Can you work these out from the model? Positions are in its coordinate system, mm. Give positions to 0.01 mm unless a question says otherwise; leave off trailing zeros. Loops run counter-clockwise (first coordinate to the right, second up) from the corner with the lowest first, then second, coordinate; pieces in that order, holes last. Notation, with made-up numbers: M 25.5,-10 L 73.5,-10 A24 cw 73.5,8 Z; hole C 42,32.5 d10. An arc over 180 degrees is marked long. Answer as a JSON object with one key per item and string values.
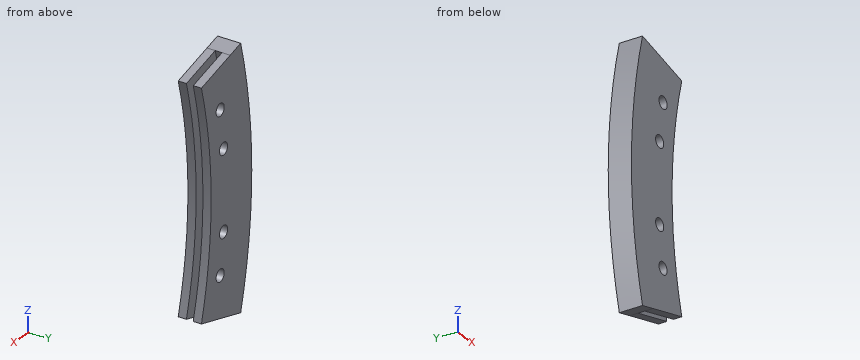
Autodesk Inventor part; units mm, degrees
ref_plane "YZ Plane" through (0, 0, 0) normal (1, 0, 0) x (0, 1, 0)
ref_plane "XZ Plane" through (0, 0, 0) normal (0, 1, 0) x (-1, 0, 0)
ref_plane "XY Plane" through (0, 0, 0) normal (0, 0, 1) x (1, 0, 0)
sketch "スケッチ1" plane through (0, 0, 0) normal (0, 1, 0) x (-1, 0, 0)
  circle A0 centre (0, 0) radius 105
  circle A1 centre (0, 0) radius 116
  line L0 (0, 0) -> (112.0474, 30.023)
  line L1 (0, 0) -> (112.0474, -30.023)
  line L2 (168, 0) -> (-168, 0)
  circle A2 centre (0, 0) radius 110 construction
  line L3 (0, 0) -> (108.3289, 19.1013) construction
  line L4 (109.5814, 9.5871) -> (0, 0) construction
  line L5 (109.5814, -9.5871) -> (0, 0) construction
  line L6 (0, 0) -> (108.3289, -19.1013) construction
  circle A3 centre (109.5814, 9.5871) radius 1.5
  circle A4 centre (108.3289, 19.1013) radius 1.5
  circle A5 centre (109.5814, -9.5871) radius 1.5
  circle A6 centre (108.3289, -19.1013) radius 1.5
  circle A7 centre (0, 0) radius 120
  line L7 (112.0474, 30.023) -> (115.9111, 31.0583)
  line L8 (112.0474, -30.023) -> (115.9111, -31.0583)
  point P0 (101.4222, -27.176)
  point P1 (101.4222, 27.176)
  dimension "d0" = 210
  dimension "d1" = 232
  dimension "d2" = 15
  dimension "d3" = 15
  dimension "d4" = 220
  dimension "d5" = 5
  dimension "d6" = 5
  dimension "d7" = 5
  dimension "d8" = 5
  dimension "d9" = 3
  dimension "d10" = 240
extrude "押し出し1" add sketch "スケッチ1" along normal blind 2 contours L2 A1 L1 A0 | A0 L0 A1 L2 | L2 A7 L8 A1 | A1 L7 A7 L2 picked at (107.2059, -25.9298) picked at (107.2059, 25.9298) picked at (115.3785, -27.3064) picked at (115.3785, 27.3064)
extrude "押し出し2" add sketch "スケッチ1" along normal blind 2.825 contours L2 A7 L8 A1 | A1 L7 A7 L2 picked at (115.3785, -27.3064) picked at (115.3785, 27.3064)
mirror "ミラー1" about plane through (-116.0237, 2.825, 0) normal (0, 1, 0)
equation "\"d6\" = d5"
equation "\"d7\" = d5"
equation "\"d8\" = d5"
properties part number "plate_cover"
1) Please list where these lines run through material, in increasing order: line 1 along Y through (x, z) = (-111, -24.5); line 2 along X through (y, z) = (1.8, 9); line 3 along Z through (x, y) = (-109, 0.3). Write a range as from..to.
Answer list:
{"line 1": "0..2, 3.65..5.65", "line 2": "-119.66..-110.96, -108.2..-104.61", "line 3": "-29.21..-20.44, -17.76..-10.97, -8.2..8.2, 10.97..17.76, 20.44..29.21"}
2) Suppose I cut it at D-D, the plane z = 21.5. Write out the boundary of the cut face in (x, y), and give its area (3 significant figures).
Answer list:
{"outline": "M -118.06,0 L -102.78,0 L -102.78,2 L -113.99,2 L -113.99,3.65 L -102.78,3.65 L -102.78,5.65 L -118.06,5.65 Z", "area": "67.8 mm^2"}
3) Suppose I cut it at A-A, the plane x = -106.25. Write out the boundary of the cut face in (y, z).
Answer list:
{"outline": "M 0,-28.47 L 2,-28.47 L 2,28.47 L 0,28.47 Z; M 3.65,-28.47 L 5.65,-28.47 L 5.65,28.47 L 3.65,28.47 Z"}
4) Suppose I cut it at B-B, the plane y = 0.65. Write out the boundary of the cut face in (x, z).
Answer list:
{"outline": "M -115.91,-31.06 L -112.05,-30.02 L -101.42,-27.18 A105 cw -101.42,27.18 L -112.05,30.02 L -115.91,31.06 A120 ccw Z; hole C -109.58,-9.59 d3; hole C -109.58,9.59 d3; hole C -108.33,-19.1 d3; hole C -108.33,19.1 d3"}
5) Will this pin go through, and if not, where does the flat tip stop? pin 1 Ø1.5 at (y, z) = (2.5, -15.5) entering from +X.
Answer list:
{"pin 1": "x = -103.76"}
6) Suppose I cut it at C-C, the plane x = -103.5. Write out the boundary of the cut face in (y, z).
Answer list:
{"outline": "M 0,-27.73 L 2,-27.73 L 2,-17.68 L 0,-17.68 Z; M 0,17.68 L 2,17.68 L 2,27.73 L 0,27.73 Z; M 3.65,-27.73 L 5.65,-27.73 L 5.65,-17.68 L 3.65,-17.68 Z; M 3.65,17.68 L 5.65,17.68 L 5.65,27.73 L 3.65,27.73 Z"}
